For this review, take the finished solid that the model builds, in its own axes (mm). Face numbers are marked on the shaded views. A direction names the side the tool comes from. Round coordinates to 2 decimals unless told otherwise and drop trailing zeros. Order: outer loops, then holes, each group sorted by start corner. A loop starts at its lowest first (then second) coordinate and runs counter-clockwise, first axis right, second up. Notation, with made-up numbers: (-15, 41) - (-9, 41) arc R28 cw to (-9, 63) - close; hole circle Ø8 at (19, -10). An arc over 180 degrees is marked (long way). One line per item, written item: value.
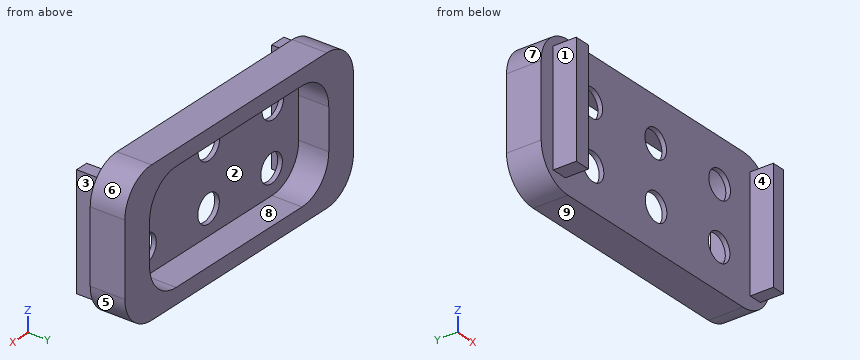
```python
from build123d import *

# Parameters (mm, degrees)
F1_DEPTH = 15
F3_DEPTH = 13
F4_R     = 6.077125
F4_R_2   = 6.056925
F5_DEPTH = 2.001
F6_W     = 6.860256
F6_H     = 48.87931
F6_W_2   = 5.716875
F7_DEPTH = 25


with BuildPart() as f1:
    # F0 (on Front) → F1 (new body)
    with BuildSketch(Plane.XZ):
        with BuildLine():
            ThreePointArc((-64.182252, -15.639039), (-59.788853, -26.245641), (-49.182252, -30.639039))
            Line((-49.182252, -30.639039), (49.182252, -30.639039))
            ThreePointArc((49.182252, -30.639039), (59.788853, -26.245641), (64.182252, -15.639039))
            Line((64.182252, -15.639039), (64.182252, 15.639039))
            ThreePointArc((64.182252, 15.639039), (59.788853, 26.245641), (49.182252, 30.639039))
            Line((49.182252, 30.639039), (-49.182252, 30.639039))
            ThreePointArc((-49.182252, 30.639039), (-59.788853, 26.245641), (-64.182252, 15.639039))
            Line((-64.182252, 15.639039), (-64.182252, -15.639039))
        make_face()
    extrude(amount=F1_DEPTH)

    # F2 (on Front) → F3 (cut)
    with BuildSketch(Plane.XZ):
        with BuildLine():
            ThreePointArc((-50.308529, -8.867968), (-45.915131, -19.47457), (-35.308529, -23.867968))
            Line((-35.308529, -23.867968), (35.308529, -23.867968))
            ThreePointArc((35.308529, -23.867968), (45.915131, -19.47457), (50.308529, -8.867968))
            Line((50.308529, -8.867968), (50.308529, 8.867968))
            ThreePointArc((50.308529, 8.867968), (45.915131, 19.47457), (35.308529, 23.867968))
            Line((35.308529, 23.867968), (-35.308529, 23.867968))
            ThreePointArc((-35.308529, 23.867968), (-45.915131, 19.47457), (-50.308529, 8.867968))
            Line((-50.308529, 8.867968), (-50.308529, -8.867968))
        make_face()
    extrude(amount=F3_DEPTH, mode=Mode.SUBTRACT)

    # F4 (on face) → F5 (cut, through all)
    with BuildSketch(Plane(origin=(0, -13, 0), x_dir=(-1, 0, 0), z_dir=(0, 1, 0))):
        with Locations((-36.016334, 11.862524)):
            Circle(F4_R)
        with Locations((-0.116334, 11.862524)):
            Circle(F4_R)
        with Locations((35.783666, 11.862524)):
            Circle(F4_R)
        with Locations((-35.730492, -13.005898)):
            Circle(F4_R_2)
        with Locations((-0.330492, -13.005898)):
            Circle(F4_R_2)
        with Locations((35.069508, -13.005898)):
            Circle(F4_R_2)
    extrude(amount=-F5_DEPTH, mode=Mode.SUBTRACT)

    # F6 (on Front) → F7 (join)
    with BuildSketch(Plane.XZ):
        with Locations((-54.024503, 0)):
            Rectangle(F6_W, F6_H)
        with Locations((56.025408, 0)):
            Rectangle(F6_W_2, F6_H)
    extrude(amount=F7_DEPTH)


solid = f1.part
```
Item 1: For P1, Ø2, axis at y = -10, z = -22, coming from the -X side; P2, Ø6, axis at x = -24, z = -13.5, coming from the -Y side; P3, Ø5, axis at x = -9.5, z = -16, coming from the +Y side, all flat-tipped, find the tip position at first contact; note any pin that passes through.
Returned:
P1: x = -63.19
P2: y = -15
P3: y = -13
Item 2: Take a section at D-D (z = -22.5). Write out the cut boundary in (x, y), plus the area to 3 significant figures.
Returned:
outline: (-62.52, -15) - (-57.45, -15) - (-57.45, -25) - (-50.59, -25) - (-50.59, -15) - (53.17, -15) - (53.17, -25) - (58.88, -25) - (58.88, -15) - (62.52, -15) - (62.52, 0) - (41.57, 0) - (41.57, -13) - (-41.57, -13) - (-41.57, 0) - (-62.52, 0) - close
area: 921 mm^2
Item 3: Take a section at C-C (x = -0.5). Write out the cut boundary in (y, z).
Returned:
outline: (-15, -30.64) - (0, -30.64) - (0, -23.87) - (-13, -23.87) - (-13, -19.01) - (-15, -19.01) - close; (-15, -7.01) - (-13, -7.01) - (-13, 5.82) - (-15, 5.82) - close; (-15, 17.91) - (-13, 17.91) - (-13, 23.87) - (0, 23.87) - (0, 30.64) - (-15, 30.64) - close
Item 4: Wall thickness on line 1 (X direction, y = -22.25, z = 22.5); line 2 (X direction, y = -14.75, z = -10.5); line 3 (Z direction, x = 27, y = -7.25): over which ranges is each line inside the solid? List them lowest first.
Returned:
line 1: -57.45 to -50.59, 53.17 to 58.88
line 2: -64.18 to -40.58, -29.56 to -5.18, 5.84 to 30.22, 41.24 to 64.18
line 3: -30.64 to -23.87, 23.87 to 30.64
Item 5: The part is to be moulded in two halves that separate along X. For the marked faces 6, 7, 8 and 9, say which applies: +X half, -X half, draft (parallel to the pull), parting line (faces both ways), or undercut.
Returned:
face 6: +X half
face 7: -X half
face 8: undercut
face 9: draft
Item 6: Take a section at B-B (y = -3). Write out the cut boundary in (x, z).
Returned:
outline: (-64.18, -15.64) arc R15 ccw to (-49.18, -30.64) - (49.18, -30.64) arc R15 ccw to (64.18, -15.64) - (64.18, 15.64) arc R15 ccw to (49.18, 30.64) - (-49.18, 30.64) arc R15 ccw to (-64.18, 15.64) - close; hole (-50.31, -8.87) arc R15 ccw to (-35.31, -23.87) - (35.31, -23.87) arc R15 ccw to (50.31, -8.87) - (50.31, 8.87) arc R15 ccw to (35.31, 23.87) - (-35.31, 23.87) arc R15 ccw to (-50.31, 8.87) - close
Item 7: Take a section at A-A (y = -20). Write out the cut boundary in (x, z), plus the area to 3 significant figures.
Returned:
outline: (-57.45, -24.44) - (-50.59, -24.44) - (-50.59, 24.44) - (-57.45, 24.44) - close; (53.17, -24.44) - (58.88, -24.44) - (58.88, 24.44) - (53.17, 24.44) - close
area: 615 mm^2
Item 8: Machinability: for the marked faces 1, 2, 3, 4 and 5, which of the approach directions +Z, -Z, +X, -X, +Y, -Y give a long, thin tool a straight path to every point of the face, cutting with its end or side? Answer none if there is none.
Returned:
face 1: +Z, -Z, -X, -Y
face 2: +Y
face 3: +Z, -Z, +X, -Y
face 4: +Z, -Z, -Y
face 5: -Z, +X, +Y, -Y
